The drawing under review shows one solid part. Ordinate dimensions are in mm from its lowest x, y, z. A direction names the side the tool comes from. Coordinates: 2 decimals unless noted, no trailing zeros. Write each loop counter-clockwise with the first axis right and the second up, starting at its lowest first coordinate (ties: lowest second). Pieces come first, ordered by that corner, then holes. Notation, with made-up numbers: M 0.5,87.5 L 33.5,87.5 A26 ccw 33.5,107.5 Z; hole C 44.25,16 d9. An arc over 180 degrees is marked long. Write each question's results on one line, items separated by ' | '. Start each with the question number.
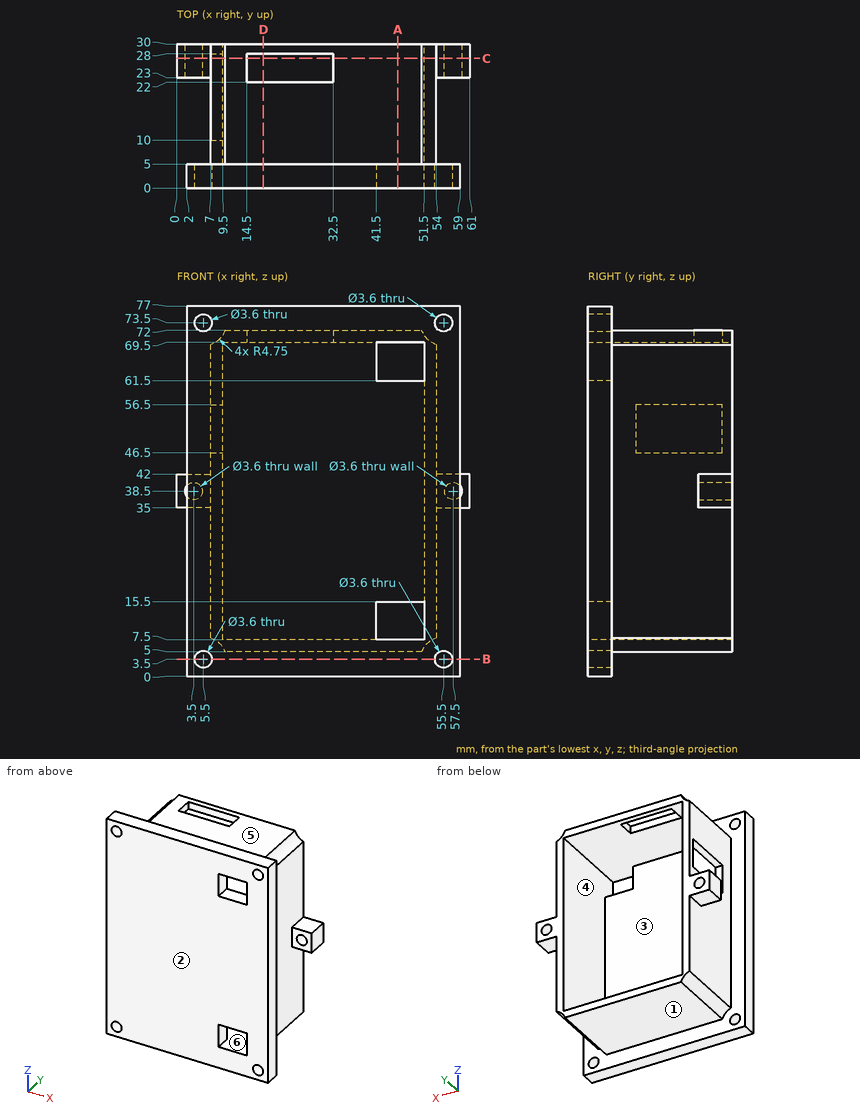
Item 1: We need section B-B on z = 3.5. State the section outline as (x, y) points.
Item 2: Draft analysis for pull direction X (two halves, no side actions). For the marked faces 4, 5 and 6, state which applies: released by +X, released by -X, zero draft, split by the parting line, or undercut.
Item 3: For the marked faces 1, 2 and 3, list the 3-axis set-ups (+Z, -Z, +X, -X, +Y, -Y) from which the entire face can be reached by the end or side of a thin tool; tool diameter is ignored.
Item 4: Insertion check: pin 1 Ø2 at (x, z) = (5.5, 73.5) entering from -Y; pin 2 Ø2 at (x, y) = (11.5, 21) entering from -Z; pin 3 Ø8 at (x, y) = (51, 18) entering from +Z; pin 4 Ø5 at (y, z) = (20.5, 49.5) entering from -X. Each pin has a flat end and moves straight along its axis. Give the tip position at first contact, or say it passes through.
Item 5: Wall thickness on L1, parallel to X at y = 25, z = 38.5; L2, parallel to Z at x = 5.5, y = 1.6; L3, parallel to X at y = 21.25, z = 59: over which ranges is each line inside the solid? List them lowest first.
Item 6: We need section A-A on x = 46. State the section outline as (y, z) points.
Item 7: We need section C-C on y = 27. Count the separate pieces of the cut face and the enclosed holes in it, then the cut area to 3 significant figures.
Item 8: We need section D-D on x = 18. State the section outline as (y, z) points.
Answer:
1) outline: M 2,0 L 3.7,0 L 3.7,5 L 2,5 Z; M 7.3,0 L 53.7,0 L 53.7,5 L 7.3,5 Z; M 57.3,0 L 59,0 L 59,5 L 57.3,5 Z
2) face 4: undercut | face 5: zero draft | face 6: undercut
3) face 1: -Z, +X, -X, +Y | face 2: +Z, -Z, +X, -X, -Y | face 3: +Y
4) pin 1: passes through | pin 2: stops at z = 5 | pin 3: stops at z = 72 | pin 4: stops at x = 51.5
5) L1: x = 0 to 1.7, 5.3 to 9.5, 51.5 to 55.7, 59.3 to 61 | L2: z = 0 to 1.7, 5.3 to 71.7, 75.3 to 77 | L3: x = 7 to 9.5, 51.5 to 54
6) outline: M 0,0 L 5,0 L 5,5 L 30,5 L 30,7.5 L 0,7.5 Z; M 0,15.5 L 5,15.5 L 5,61.5 L 0,61.5 Z; M 0,69.5 L 30,69.5 L 30,72 L 5,72 L 5,77 L 0,77 Z
7) separate pieces: 2 | enclosed holes: 2 | area: 529 mm^2
8) outline: M 0,0 L 5,0 L 5,5 L 30,5 L 30,7.5 L 5,7.5 L 5,69.5 L 22,69.5 L 22,72 L 5,72 L 5,77 L 0,77 Z; M 28,69.5 L 30,69.5 L 30,72 L 28,72 Z
